```python
from build123d import *

# Parameters (mm, degrees)
F1_DEPTH = 3.175
F0_W     = 30.48
F0_H     = 32.512
F2_DEPTH = 12.192


with BuildPart() as f1:
    # F0 (on Front) → F1 (new body)
    with BuildSketch(Plane.XZ):
        Polygon((-11.6948662326, 48.9731033504), (-76.444491744, 48.9731033504), (-76.444491744, -52.6268966496), (-11.6948662326, -52.6268966496), (-11.6948662326, -20.1148966496), (18.7851337674, -20.1148966496), (18.7851337674, -52.6268966496), (75.955508256, -52.6268966496), (75.955508256, -15.5456149951), (22.8138189573, -15.5456149951), (-24.9381810427, -15.5456149951), (-24.9381810427, 9.8543850049), (22.8138189573, 9.8543850049), (22.8138189573, 48.9731033504), (18.7851337674, 48.9731033504), (18.7851337674, 16.4611033504), (-11.6948662326, 16.4611033504), align=None)
    extrude(amount=-F1_DEPTH)

    # F0 (on Front) → F2 (join)
    with BuildSketch(Plane.XZ):
        with Locations((3.5451337674, 32.7171033504)):
            Rectangle(F0_W, F0_H)
        with Locations((3.5451337674, -36.3708966496)):
            Rectangle(F0_W, F0_H)
    extrude(amount=-F2_DEPTH)


solid = f1.part
```
The model under review builds one solid part; all positions refer to its coordinate system, in mm. A direction names the side the tool comes from. Give positions to 0.01 mm unless a question says otherwise; leave off trailing zeros. Write each loop counter-clockwise with the first axis right and the second up, starting at its lowest first coordinate (ties: lowest second). Pieces come first, ordered by that corner, then holes.
(1) Consider section C-C, the plane z = 29. Give the boundary of the cut face in (x, y) (1 decimal), and give its area (3 significant figures).
(2) Consider section D-D, the plane x = -33. Give the boundary of the cut face in (y, z) (3 decimals).
(3) Consider section B-B, the plane y = 10. Give the boundary of the cut face in (x, z).
(4) To check wall thickness, follow L1, parallel to Z at x = 8, y = 4.5; L2, parallel to Y at x = -28.5, z = 41.5 (3 decimals); L3, parallel to Z at x = 15, y = 2. State the ranges of each line that lie inside material, in increasing order.
(5) The part is to be moulded in two halves that separate along Z. For faces 5 (the flat face through (26, 2, -15.546)), 6 (the flat face through (-5, 5, 48.973)), 7 (the flat face through (18.785, 8, -37)), 8 (the flat face through (3, 8, -20.115)), say which applies: released by +Z, released by -Z, zero draft, split by the parting line, or undercut.
(6) Tool access review of faces 1 (the flat face through (-1, 2, 9.854)), 2 (the flat face through (18.785, 8, 32)), 3 (the flat face through (3, 8, 16.461)), 4 (the flat face through (-11.695, 8, 32)): name each direction out of +Z, -Z, +X, -X, +Y, -Y from which nothing blocks a thin tool from reaching the whole face with its end or side.
(7) For P1, Ø4.5, axis at y = 7, z = -42.5, coming from the -X side; P2, Ø3, axis at y = 5, z = -14.5, coming from the +X side; P3, Ø1.6, axis at y = 2, z = -5.5, coming from the +X side; P4, Ø3.5, axis at x = 25.5, y = 1.5, coming from the +Z side, all flat-tipped, find the tip position at first contact; note any pin that passes through.
(8) Consider section A-A, the plane x = 1.5. Give the boundary of the cut face in (y, z) (3 decimals).
Returned:
1. outline: (-76.4, 0) - (22.8, 0) - (22.8, 3.2) - (18.8, 3.2) - (18.8, 12.2) - (-11.7, 12.2) - (-11.7, 3.2) - (-76.4, 3.2) - close
1. area: 590 mm2
2. outline: (0, -52.627) - (3.175, -52.627) - (3.175, 48.973) - (0, 48.973) - close
3. outline: (-11.69, -52.63) - (18.79, -52.63) - (18.79, -20.11) - (-11.69, -20.11) - close; (-11.69, 16.46) - (18.79, 16.46) - (18.79, 48.97) - (-11.69, 48.97) - close
4. L1: z = -52.63 to -20.11, 16.46 to 48.97
4. L2: y = 0 to 3.175
4. L3: z = -52.63 to -15.55, 9.85 to 48.97
5. face 5: undercut
5. face 6: released by +Z
5. face 7: zero draft
5. face 8: undercut
6. face 1: +X, +Y, -Y
6. face 2: +Z, -Z, +X, +Y
6. face 3: +X, -X, +Y
6. face 4: +Z, -Z, -X, +Y
7. P1: stops at x = -11.69
7. P2: passes through
7. P3: stops at x = -24.94
7. P4: stops at z = -15.55
8. outline: (0, -52.627) - (12.192, -52.627) - (12.192, -20.115) - (3.175, -20.115) - (3.175, -15.546) - (0, -15.546) - close; (0, 9.854) - (3.175, 9.854) - (3.175, 16.461) - (12.192, 16.461) - (12.192, 48.973) - (0, 48.973) - close
